from build123d import *

# Parameters (mm, degrees)
SKETCH_1_W          = 60
SKETCH_1_H          = 20
EXTRUDE_1_DEPTH     = 2
SKETCH_2_W          = 20
SKETCH_2_H          = 16
CUT_EXTRUDE_1_DEPTH = 64.277168078
FILLET_1_R          = 1
SKETCH_3_R          = 2.25
CUT_EXTRUDE_2_DEPTH = 64.277168078
SKETCH_4_W          = 36
SKETCH_4_H          = 20
CUT_EXTRUDE_3_DEPTH = 10


with BuildPart() as part:
    # 草图1 → 凸台-拉伸1 (new body)
    with BuildSketch(Plane.XY):
        with Locations((30, 10)):
            Rectangle(SKETCH_1_W, SKETCH_1_H)
    extrude(amount=EXTRUDE_1_DEPTH)

    # 草图2 → 切除-拉伸1 (cut, through all)
    with BuildSketch(Plane.XY.offset(2)):
        with Locations((30, 8)):
            Rectangle(SKETCH_2_W, SKETCH_2_H)
    extrude(amount=-CUT_EXTRUDE_1_DEPTH, mode=Mode.SUBTRACT)

    # 圆角1
    fillet_1_edges = [part.edges().sort_by_distance(p)[0] for p in [
        (20, 16, 1),
        (40, 16, 1),
    ]]
    fillet(fillet_1_edges, radius=FILLET_1_R)

    # 草图3 → 切除-拉伸2 (cut, through all)
    with BuildSketch(Plane.XY.offset(2)):
        with Locations((7, 15)):
            Circle(SKETCH_3_R)
        with Locations(Location((53, 15, 0), (0, 0, 180))):
            Circle(SKETCH_3_R)
        with Locations((53, 5)):
            Circle(SKETCH_3_R)
        with Locations(Location((7, 5, 0), (0, 0, 180))):
            Circle(SKETCH_3_R)
    extrude(amount=-CUT_EXTRUDE_2_DEPTH, mode=Mode.SUBTRACT)

    # 草图4 → 切除-拉伸3 (cut)
    with BuildSketch(Plane.XY.offset(2)):
        with Locations((42, 10)):
            Rectangle(SKETCH_4_W, SKETCH_4_H)
    extrude(amount=-CUT_EXTRUDE_3_DEPTH, mode=Mode.SUBTRACT)


solid = part.part
Input: part model. Units: mm. Frame: model coordinates. A direction names the side the tool comes from. Round coordinates to 2 decimals unless told otherwise and drop trailing zeros. Order: outer loops, then holes, each group sorted by start corner. A loop starts at its lowest first (then second) coordinate and runs counter-clockwise, first axis right, second up. Notation, with made-up numbers: (12, -3) - (51, -3) arc R14 ccw to (51, 4) - close; hole circle Ø6 at (28, -39.5). An arc over 180 degrees is marked (long way). Use a Markdown table: item, result.
1. Section B-B on x = 7. Return the cut outline in (y, z), then the cut area to 3 significant figures.
Evaluation:
| item | result |
|---|---|
| outline | (0, 0) - (2.75, 0) - (2.75, 2) - (0, 2) - close; (7.25, 0) - (12.75, 0) - (12.75, 2) - (7.25, 2) - close; (17.25, 0) - (20, 0) - (20, 2) - (17.25, 2) - close |
| area | 22.0 mm^2 |
2. Section C-C on z = 1.2. Return the cut outline in (x, y).
Evaluation:
| item | result |
|---|---|
| outline | (0, 0) - (20, 0) - (20, 15) arc R1 cw to (21, 16) - (24, 16) - (24, 20) - (0, 20) - close; hole circle Ø4.5 at (7, 5); hole circle Ø4.5 at (7, 15) |
3. Section D-D on y = 1.5. Return the cut outline in (x, z), then the cut area to 3 significant figures.
Evaluation:
| item | result |
|---|---|
| outline | (0, 0) - (20, 0) - (20, 2) - (0, 2) - close |
| area | 40.0 mm^2 |
4. Access query for faces 4 (the face through (24, 18, 1)), 5 (the face through (20, 7, 1)). Directions: +Z, -Z, +X, -X, +Y, -Y. A direction counts if a zero-diameter tool reaches every point of the face in a straight line with its end or side. Return the directions, or none.
Evaluation:
| item | result |
|---|---|
| face 4 | +Z, -Z, +X, +Y, -Y |
| face 5 | +Z, -Z, +X, -Y |
5. Mould query, pull axis Y, two halves, no side actions, for faces 1 (the face through (12, 20, 1)), 2 (the face through (6.512, 12.804, 1.014)), 3 (the face through (22, 16, 1)). Classes: +Y half, -Y half, draft (parallel to the pull), parting line (faces both ways), or undercut.
Evaluation:
| item | result |
|---|---|
| face 1 | +Y half |
| face 2 | undercut |
| face 3 | -Y half |
6. Material intervals for probe 1 along Y at (x, z) = (7, 1.35); probe 2 along X at (y, z) = (5, 1); probe 3 along X at (y, z) = (9.75, 1.2), sorted ascending.
Evaluation:
| item | result |
|---|---|
| probe 1 | 0 to 2.75, 7.25 to 12.75, 17.25 to 20 |
| probe 2 | 0 to 4.75, 9.25 to 20 |
| probe 3 | 0 to 20 |
7. First-contact query: pin 1 (2 mm diameter, centred on x = 13.5, y = 6.5, fed in from -Z); pin 2 (0.6 mm diameter, centred on x = 23, z = 1, fed in from -Y). Flat tips, straight axial feed; report the tip coordinate or a pass-through.
Evaluation:
| item | result |
|---|---|
| pin 1 | z = 0 |
| pin 2 | y = 16 |
8. Section A-A on y = 5. Return the cut outline in (x, z), then the cut area to 3 significant figures.
Evaluation:
| item | result |
|---|---|
| outline | (0, 0) - (4.75, 0) - (4.75, 2) - (0, 2) - close; (9.25, 0) - (20, 0) - (20, 2) - (9.25, 2) - close |
| area | 31.0 mm^2 |
